from build123d import *

# Parameters (mm, degrees)
SKETCH1_W           = 55
SKETCH1_H           = 78.5
BOSS_EXTRUDE1_DEPTH = 2.5
SKETCH6_W           = 55
SKETCH6_H           = 10
BOSS_EXTRUDE2_DEPTH = 16.3
CUT_EXTRUDE1_DEPTH  = 71.135600803
SKETCH9_W           = 55
SKETCH9_H           = 12
BOSS_EXTRUDE3_DEPTH = 5
CUT_EXTRUDE4_DEPTH  = 5
CUT_EXTRUDE2_DEPTH  = 2.5
BOSS_EXTRUDE4_DEPTH = 65
FILLET1_R           = 0.5
CUT_EXTRUDE3_DEPTH  = 5
FILLET2_R           = 3


with BuildPart() as part:
    # Sketch1 → Boss-Extrude1 (new, symmetric)
    with BuildSketch(Plane(origin=(0, 0, 0), x_dir=(0, 0, -1), z_dir=(1, 0, 0))):
        Rectangle(SKETCH1_W, SKETCH1_H)
        with BuildLine():
            Line((-1.7, -32.75), (-1.7, -12.75))
            ThreePointArc((-1.7, -12.75), (0, -11.05), (1.7, -12.75))
            Line((1.7, -12.75), (1.7, -32.75))
            ThreePointArc((1.7, -32.75), (0, -34.45), (-1.7, -32.75))
        make_face(mode=Mode.SUBTRACT)
        with BuildLine():
            Line((-1.7, 32.75), (-1.7, 12.75))
            ThreePointArc((-1.7, 12.75), (0, 11.05), (1.7, 12.75))
            Line((1.7, 12.75), (1.7, 32.75))
            ThreePointArc((1.7, 32.75), (0, 34.45), (-1.7, 32.75))
        make_face(mode=Mode.SUBTRACT)
    extrude(amount=BOSS_EXTRUDE1_DEPTH, both=True)

    # Sketch6 → Boss-Extrude2 (add)
    with BuildSketch(Plane.ZY.offset(2.5)):
        Rectangle(SKETCH6_W, SKETCH6_H)
    extrude(amount=BOSS_EXTRUDE2_DEPTH)

    # Sketch7 → Cut-Extrude1 (cut, through all)
    with BuildSketch(Plane.XY.offset(27.5)):
        with BuildLine():
            Line((-15.05, 5), (-18.8, 5))
            Line((-18.8, 5), (-18.8, -5))
            Line((-18.8, -5), (-15.05, -5))
            ThreePointArc((-15.05, -5), (-12.55, 0), (-15.05, 5))
        make_face()
    extrude(amount=-CUT_EXTRUDE1_DEPTH, mode=Mode.SUBTRACT)

    # Sketch9 → Boss-Extrude3 (add)
    with BuildSketch(Plane.ZY.offset(2.5)):
        with Locations((0, 45.25)):
            Rectangle(SKETCH9_W, SKETCH9_H)
    boss_extrude3 = extrude(amount=-BOSS_EXTRUDE3_DEPTH)

    # Sketch16 → Cut-Extrude4 (cut)
    with BuildSketch(Plane.ZY.offset(2.5)):
        Polygon((10.25, 51.25), (17.25, 51.25), (18.75, 46.25), (8.75, 46.25), align=None)
        Polygon((-18.75, 46.25), (-8.75, 46.25), (-10.25, 51.25), (-17.25, 51.25), align=None)
    cut_extrude4 = extrude(amount=-CUT_EXTRUDE4_DEPTH, mode=Mode.SUBTRACT)

    # Mirror1: Boss-Extrude3 across plane
    add(boss_extrude3.mirror(Plane.ZX))

    # Sketch10 → Cut-Extrude2 (cut)
    with BuildSketch(Plane(origin=(0, 0, 0), x_dir=(0, 0, -1), z_dir=(1, 0, 0))):
        with BuildLine():
            Line((3.25, -18.75), (3.25, -26.75))
            ThreePointArc((3.25, -26.75), (0, -30), (-3.25, -26.75))
            Line((-3.25, -26.75), (-3.25, -18.75))
            ThreePointArc((-3.25, -18.75), (0, -15.5), (3.25, -18.75))
        make_face()
        with BuildLine():
            Line((3.25, 18.75), (3.25, 26.75))
            ThreePointArc((3.25, 26.75), (0, 30), (-3.25, 26.75))
            Line((-3.25, 26.75), (-3.25, 18.75))
            ThreePointArc((-3.25, 18.75), (0, 15.5), (3.25, 18.75))
        make_face()
    extrude(amount=-CUT_EXTRUDE2_DEPTH, mode=Mode.SUBTRACT)

    # Sketch11 → Boss-Extrude4 (add)
    with BuildSketch(Plane(origin=(0, 0, -27.5), x_dir=(-1, 0, 0), z_dir=(0, 0, -1))):
        with BuildLine():
            Line((-2.5, -13), (2.5, -13))
            Line((2.5, -13), (2.5, -5))
            Line((2.5, -5), (15.05, -5))
            ThreePointArc((15.05, -5), (12.55, 0), (15.05, 5))
            Line((15.05, 5), (2.5, 5))
            Line((2.5, 5), (2.5, 13))
            Line((2.5, 13), (-2.5, 13))
            Line((-2.5, 13), (-2.5, -13))
        make_face()
    extrude(amount=BOSS_EXTRUDE4_DEPTH)

    # Fillet1
    fillet1_edges = [part.edges().sort_by_distance(p)[0] for p in [
        (-15.05, 5, -32.5),
        (-15.05, -5, -32.5),
    ]]
    fillet(fillet1_edges, radius=FILLET1_R)

    # Sketch15 → Cut-Extrude3 (cut)
    with BuildSketch(Plane.ZY.offset(2.5)):
        Polygon((-40.25, 13), (-38.75, 8), (-48.75, 8), (-47.25, 13), align=None)
        Polygon((-72.75, 13), (-79.75, 13), (-81.25, 8), (-71.25, 8), align=None)
    cut_extrude3 = extrude(amount=-CUT_EXTRUDE3_DEPTH, mode=Mode.SUBTRACT)

    # Mirror2: Cut-Extrude3 across plane
    add(cut_extrude3.mirror(Plane.ZX), mode=Mode.SUBTRACT)

    # Mirror3: Cut-Extrude4 across plane
    add(cut_extrude4.mirror(Plane.ZX), mode=Mode.SUBTRACT)

    # Fillet2
    fillet2_edges = [part.edges().sort_by_distance(p)[0] for p in [
        (0, -51.25, 27.5),
        (0, -51.25, -27.5),
        (0, 13, -27.5),
        (0, -13, -27.5),
        (0, 13, -92.5),
        (0, -13, -92.5),
        (0, 51.25, -27.5),
        (0, 51.25, 27.5),
    ]]
    fillet(fillet2_edges, radius=FILLET2_R)


solid = part.part
The listing builds one solid part. Answer for the finished solid, in the listing's coordinates (mm). A direction names the side the tool comes from. Give positions to 0.01 mm unless a question says otherwise; leave off trailing zeros. Write each loop counter-clockwise with the first axis right and the second up, starting at its lowest first coordinate (ties: lowest second). Pieces come first, ordered by that corner, then holes.
Item 1: Which of the six approach directions +Z, -Z, +X, -X, +Y, -Y give full straight-line access (tool end or side, diameter ignored) to faces 4 (the flat face through (0, 10.5, -72)), 5 (the cylindrical face through (-1, 28, 3)), 6 (the flat face through (0, 32, -27.5)), 7 (the flat face through (0, 51.25, 0))?
Item 2: Find the intervals of material crossed by line 1 along X through (y, z) = (-46, -26); line 2 along Z through (x, y) = (1.75, 40); line 3 along Y through (x, z) = (-8, -6), in increasing order.
Item 3: Determine the mould class of faces 1 (the flat face through (0, 10.5, -80.5)), 2 (the flat face through (0, 13, -85)), 3 (the flat face through (0, -13, -60)) for opening direction Y: released by +Y, released by -Y, zero draft, split by the parting line, or undercut.
Item 4: Flat-ended cylindrical pins translate along their axes: P1, Ø1.5, axis at x = -1, z = -11.5, coming from the -Y side; P2, Ø0.5, axis at y = -25.5, z = 2.5, coming from the -X side; P3, Ø1.5, axis at x = 1, y = -18, coming from the -Z side; P4, Ø3, axis at x = -10.5, y = 8, coming from the +Z side. Find the tip coordinate at first contact, or state that the pin passes through.
Item 5: Section B-B, the plane y = -40 is taken. Write down the section's boundary in (x, z), plus the area to 3 significant figures.
Item 6: Section C-C, the plane x = -10.75 is taken. Write down the section's boundary in (y, z).
Item 7: Section A-A, the plane z = 0 is taken. Write down the section's boundary in (x, y), plus the area to 3 significant figures.
Completed:
1. face 4: +X, -X
1. face 5: -X
1. face 6: -Z, +X, -X, +Y
1. face 7: +Z, -Z, +X, -X, +Y
2. line 1: x = -2.5 to 2.5
2. line 2: z = -27.5 to 27.5
2. line 3: y = -5 to 5
3. face 1: undercut
3. face 2: released by +Y
3. face 3: released by -Y
4. P1: stops at y = -46.25
4. P2: stops at x = 0
4. P3: stops at z = -27.5
4. P4: passes through
5. outline: (-2.5, -27.5) - (2.5, -27.5) - (2.5, 27.5) - (-2.5, 27.5) - close
5. area: 275 mm2
6. outline: (-5, -92.5) - (5, -92.5) - (5, 27.5) - (-5, 27.5) - close
7. outline: (-14.14, -4.17) arc R0.5 ccw to (-13.77, -5) - (-2.5, -5) - (-2.5, -11.05) - (2.5, -11.05) - (2.5, 11.05) - (-2.5, 11.05) - (-2.5, 5) - (-13.77, 5) arc R0.5 ccw to (-14.14, 4.17) arc R6.25 cw to start; (-2.5, -51.25) - (2.5, -51.25) - (2.5, -34.45) - (-2.5, -34.45) - close; (-2.5, 34.45) - (2.5, 34.45) - (2.5, 51.25) - (-2.5, 51.25) - close
7. area: 386 mm2
